Can you work these out from the model? Positions are in its coordinate system, mm. A direction names the side the tool comes from. Round coordinates to 2 decimals unless told otherwise and drop trailing zeros. Order: outer loops, then holes, each group sorted by start corner. A loop starts at its lowest first (then second) coordinate and runs counter-clockwise, first axis right, second up. Notation, with made-up numbers: M 36,74 L 87,74 A23 cw 87,83 Z; hole C 81,45 d1. An arc over 180 degrees is marked long. Answer as a JSON object with one key per item and string values. Group by question number.
from build123d import *
from OCP.BRepFilletAPI import BRepFilletAPI_MakeFillet

# Parameters (mm, degrees)
SKETCH1_W           = 3.05
SKETCH1_H           = 2.41
BOSS_EXTRUDE1_DEPTH = 8.51
CUT_EXTRUDE1_START  = 8.51
SKETCH1_3_W         = 0.64
SKETCH1_3_H         = 0.64
CUT_EXTRUDE1_DEPTH  = 5
CHAMFER1_SIZE       = 0.5
BOSS_EXTRUDE2_DEPTH = 0.32
FILLET1_R1          = 0.5
FILLET1_R2          = 1.14
CHAMFER2_SIZE       = 0.2


with BuildPart() as part:
    # Sketch1 → Boss-Extrude1 (new body)
    with BuildSketch(Plane.XY):
        Rectangle(SKETCH1_W, SKETCH1_H)
    extrude(amount=BOSS_EXTRUDE1_DEPTH)

    # Sketch1<3> → Cut-Extrude1 (cut)
    with BuildSketch(Plane.XY.offset(CUT_EXTRUDE1_START)):
        Rectangle(SKETCH1_3_W, SKETCH1_3_H)
    extrude(amount=-CUT_EXTRUDE1_DEPTH, mode=Mode.SUBTRACT)

    # Chamfer1
    chamfer1_edges = [part.edges().sort_by_distance(p)[0] for p in [
        (-0.32, 0, 8.51),
        (0, -0.32, 8.51),
        (0.32, 0, 8.51),
        (0, 0.32, 8.51),
    ]]
    chamfer(chamfer1_edges, length=CHAMFER1_SIZE)

    # Sketch2 → Boss-Extrude2 (add, symmetric)
    with BuildSketch(Plane(origin=(0, 0, 0), x_dir=(0, 0, -1), z_dir=(1, 0, 0))):
        Polygon((0, -0.32), (1.2, -0.32), (1.2, -3.745), (1.84, -3.745), (1.84, 0.32), (0, 0.32), align=None)
    extrude(amount=BOSS_EXTRUDE2_DEPTH, both=True)

    # Fillet1: one fillet with a radius per group of edges: ONE call of the kernel's fillet builder (fillet() takes one radius for all edges)
    fillet1_edges_1 = [part.edges().sort_by_distance(p)[0] for p in [
        (0, -0.32, -1.2),
    ]]
    fillet1_edges_2 = [part.edges().sort_by_distance(p)[0] for p in [
        (0, 0.32, -1.84),
    ]]
    fillet1 = BRepFilletAPI_MakeFillet(part.part.solid().wrapped)
    for e in fillet1_edges_1:
        fillet1.Add(FILLET1_R1, e.wrapped)
    for e in fillet1_edges_2:
        fillet1.Add(FILLET1_R2, e.wrapped)
    add(Compound.cast(fillet1.Shape()), mode=Mode.REPLACE)

    # Chamfer2
    chamfer2_edges = [part.edges().sort_by_distance(p)[0] for p in [
        (-0.32, -3.745, -1.52),
        (0, -3.745, -1.2),
        (0, -3.745, -1.84),
        (0.32, -3.745, -1.52),
    ]]
    chamfer(chamfer2_edges, length=CHAMFER2_SIZE)


solid = part.part
Item 1: I'm going to push flat-ended pins straight in: pin 1 Ø0.7 at (x, y) = (-0.5, 0) entering from -Z; pin 2 Ø0.5 at (x, z) = (0, -0.5) entering from +Y; pin 3 Ø1 at (x, z) = (-0.5, 2) entering from -Y (3 decimals). Where does each tip first touch, or does it pass through?
Item 2: Suppose I cut it at A-A, the plane y = -0.95. Write out the boundary of the cut face in (x, z) (3 decimals), and give its area (3 significant figures).
Item 3: Suppose I cut it at C-C, the plane x = -0.7. Write out the boundary of the cut face in (y, z) (3 decimals).
Item 4: Suppose I cut it at B-B, the plane z = 7.5. Write out the boundary of the cut face in (x, y) (3 decimals).
Item 5: I need wall thicknesses on line 1 (X direction, y = 0.15, z = 5) (3 decimals); line 2 (Y direction, x = -0.2, z = 7.5) (3 decimals); line 3 (Z direction, x = -0.1, y = -2.55). Which ranges of each line are inside material? Lowest first, please.
Item 6: Suppose I cut it at D-D, the plane y = 0.65. Write out the boundary of the cut face in (x, z) (3 decimals).
Item 7: On a 3-axis mill with a long thin cutter (end or side, diameter ignored), from which of +Z, -Z, +X, -X, +Y, -Y can I reach the whole of each face in a straight line? I mean faces 1 (the face through (0.32, -1.2, -1.5)), 2 (the face through (-0.32, -1.2, -1.5)), 3 (the face through (0, 1.205, 4)), 4 (the face through (0, -1.205, 4)). Say none if no direction works.
Computed:
{
 "1": {"pin 1": "stops at z = -1.71", "pin 2": "stops at y = 0.32", "pin 3": "stops at y = -1.205"},
 "2": {"outline": "M -1.525,0 L 1.525,0 L 1.525,8.51 L -1.525,8.51 Z; M -0.32,-1.84 L 0.32,-1.84 L 0.32,-1.2 L -0.32,-1.2 Z", "area": "26.4 mm^2"},
 "3": {"outline": "M -1.205,0 L 1.205,0 L 1.205,8.51 L 0.82,8.51 L 0.7,8.39 L -0.7,8.39 L -0.82,8.51 L -1.205,8.51 Z"},
 "4": {"outline": "M -1.525,-1.205 L 1.525,-1.205 L 1.525,1.205 L -1.525,1.205 Z; hole M -0.32,-0.32 L 0.32,-0.32 L 0.32,0.32 L -0.32,0.32 Z"},
 "5": {"line 1": "x = -1.525 to -0.32, 0.32 to 1.525", "line 2": "y = -1.205 to -0.32, 0.32 to 1.205", "line 3": "z = -1.84 to -1.2"},
 "6": {"outline": "M -1.525,0 L 1.525,0 L 1.525,8.51 L 0.82,8.51 L 0.65,8.34 L -0.65,8.34 L -0.82,8.51 L -1.525,8.51 Z"},
 "7": {"face 1": "-Z, +X, +Y, -Y", "face 2": "-Z, -X, +Y, -Y", "face 3": "+Z, -Z, +X, -X, +Y", "face 4": "+Z, +X, -X, -Y"}
}
